The figure shows three views and two pictorial views of one solid part (mm, origin at its lowest corner). Answer the questions. Round coordinates to 2 decimals unless told otherwise and drop trailing zeros. Order: outer loops, then holes, each group sorted by start corner. A loop starts at its lowest first (then second) coordinate and runs counter-clockwise, first axis right, second up. Notation, with made-up numbers: M -34.75,71.5 L 24.25,71.5 A20 cw 24.25,83.5 Z; hole C 78,20.25 d10. An arc over 180 degrees is marked long. Answer as CSV lines item,"result".
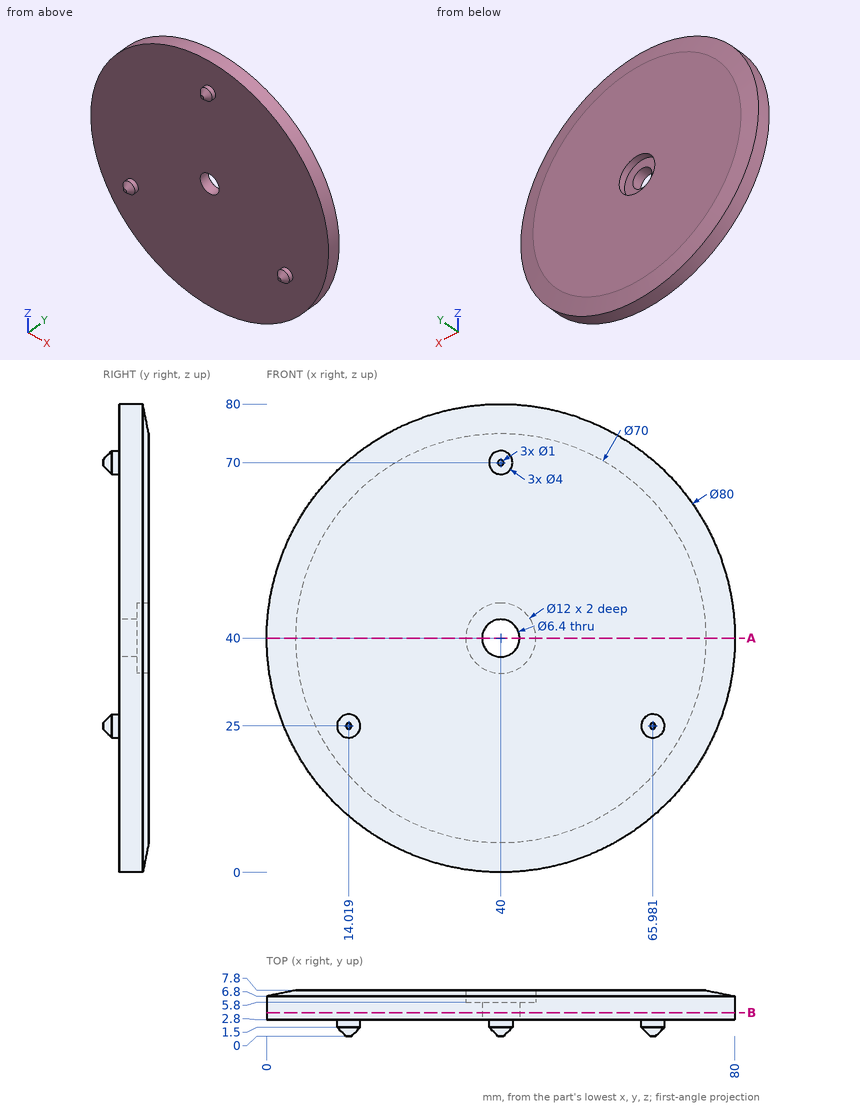
Item 1: A cutting plane is placed at B-B, the plane y = 4. Determine the outline of the cut face in (x, z), and give its area (3 significant figures).
Ans:
outline,"C 40,40 d80; hole C 40,40 d6.4"
area,"4,990 mm2"
Item 2: A cutting plane is placed at A-A, the plane z = 40. Determine the outline of the cut face in (x, y).
Ans:
outline,"M 0,2.8 L 36.8,2.8 L 36.8,5.8 L 34,5.8 L 34,7.8 L 5,7.8 L 0,6.8 Z; M 43.2,2.8 L 80,2.8 L 80,6.8 L 75,7.8 L 46,7.8 L 46,5.8 L 43.2,5.8 Z"
Item 3: Find the intervals of material crossed by probe 1 along X at (y, z) = (3.8, 40); probe 2 along Y at (x, z) = (40, 19.5); probe 3 along Z at (x, y) = (39, 4.25), in increasing order. Write a range as [from, to].
Ans:
probe 1,"[0, 36.8], [43.2, 80]"
probe 2,"[2.8, 7.8]"
probe 3,"[0.01, 36.96], [43.04, 79.99]"
Item 4: Flat-ended cylindrical pins translate along their axes: pin 1 (1.5 mm diameter, centred on x = 43, y = 6, fed in from +Z); pin 2 (24 mm diameter, centred on x = 45, z = 48.5, fed in from -Y); pin 3 (1.5 mm diameter, centred on x = 27, y = 3.5, fed in from +Z); pin 4 (9.5 mm diameter, centred on x = 39.5, z = 43, fed in from +Y). Find the tip coordinate at first contact, or state that the pin passes through.
Ans:
pin 1,"z = 79.94"
pin 2,"y = 2.8"
pin 3,"z = 78.08"
pin 4,"y = 7.8"
